Autodesk Inventor part; units mm, degrees
ref_plane "YZ Plane" through (0, 0, 0) normal (1, 0, 0) x (0, 1, 0)
ref_plane "XZ Plane" through (0, 0, 0) normal (0, 1, 0) x (-1, 0, 0)
ref_plane "XY Plane" through (0, 0, 0) normal (0, 0, 1) x (1, 0, 0)
sketch "Skizze1" plane through (0, 0, 0) normal (0, 1, 0) x (-1, 0, 0)
  circle A0 centre (0, 0) radius 27
  circle A1 centre (0, 0) radius 30
  dimension "d0" = 54
  dimension "d10" = 60
extrude "Extrusion1" add sketch "Skizze1" along normal blind 190
sketch "Skizze4" plane through (0, 0, 0) normal (0, -1, 0) x (1, 0, 0)
  circle A0 centre (0, 0) radius 30
  point P0 (0, 30)
  point P1 (-25.9808, -15)
  point P2 (25.9808, -15)
  dimension "d11" = 30
  dimension "d14" = 360
ref_plane "Arbeitsebene2" through (0, 0, 30) normal (0, 0, 1) x (1, 0, 0)
ref_plane "Arbeitsebene3" through (25.9808, 0, -15) normal (0.866, 0, -0.5) x (0, 1, 0)
ref_plane "Arbeitsebene4" through (-25.9808, 0, -15) normal (-0.866, 0, -0.5) x (0, -1, 0)
sketch "Skizze5" plane through (25.9808, 0, -15) normal (0.866, 0, -0.5) x (0, 1, 0)
  line L0 (0, 30) -> (0, -30)
  line L1 (0, 30) -> (190, 30)
  point P0 (0, 0)
  point P1 (50, 0)
  point P2 (140, 0)
  dimension "d16" = 50
  dimension "d17" = 90
  dimension "d18" = 30
  dimension "d19" = 30
sketch "Skizze6" plane through (0, 0, 30) normal (0, 0, 1) x (1, 0, 0)
  line L0 (-30, 0) -> (-30, 190)
  line L1 (-30, 0) -> (30, 0)
  point P0 (0, 0)
  point P1 (0, 20)
  point P2 (0, 110)
  dimension "d20" = 90
  dimension "d21" = 30
  dimension "d22" = 30
  dimension "d23" = 20
sketch "Skizze7" plane through (-25.9808, 0, -15) normal (-0.866, 0, -0.5) x (0, -1, 0)
  line L0 (0, 30) -> (-190, 30)
  point P0 (0, 0)
  point P1 (-80, 0)
  point P2 (-170, 0)
  dimension "d24" = 30
  dimension "d25" = 80
  dimension "d47" = 90
  dimension "d48" = 30
hole "Bohrung1" at (-25.9808, 80, -15) at (-25.9808, 170, -15) direction (0.866, 0, 0.5) diameter 3.3 depth 8 tip angle 118
hole "Bohrung2" at (0, 110, 30) at (0, 20, 30) direction (0, 0, -1) diameter 3.3 depth 8 tip angle 118
hole "Bohrung3" at (25.9808, 50, -15) at (25.9808, 140, -15) direction (-0.866, 0, 0.5) diameter 3.3 depth 8 tip angle 118
properties part number "cylinder"
Build history of the part. All positions in model axes, mm. A direction names the side the tool comes from. Give positions to 0.01 mm unless a question says otherwise; leave off trailing zeros. Order: outer loops, then holes, each group sorted by start corner. A loop starts at its lowest first (then second) coordinate and runs counter-clockwise, first axis right, second up. Notation, with made-up numbers: M -25.75,66 L -1.75,66 A16 ccw -1.75,86 Z; hole C -2.75,28 d10. An arc over 180 degrees is marked long. Use one line per item in the form item = value.
Q1. Wall check: probe 1 along Y at (x, z) = (0, 29); probe 2 along Z at (x, y) = (0, 68); probe 3 along Z at (x, y) = (6.5, 74.5). Give the ranges that are in metal, low to high.
Conclusion:
probe_1 = 0 to 18.35, 21.65 to 108.35, 111.65 to 190
probe_2 = -30 to -27, 27 to 30
probe_3 = -29.29 to -26.21, 26.21 to 29.29
Q2. Pin check, flat tips, straight feed: P1, Ø4, axis at y = 74.5, z = 9.5, coming from the +X side; P2, Ø8, axis at y = 54, z = 8, coming from the -X side; P3, Ø10, axis at y = 158, z = -16, coming from the -X side. Stop position of each tip, or through.
Conclusion:
P1 = 29.05
P2 = -29.73
P3 = -27.91
Q3. Slice it at B-B, the plane z = 17.5. Write the cut outline in (x, y).
Conclusion:
outline = M -24.37,0 L -20.56,0 L -20.56,190 L -24.37,190 Z; M 20.56,0 L 24.37,0 L 24.37,190 L 20.56,190 Z
Q4. Slice it at C-C, the plane y = 44.5. Write the cut outline in (x, z).
Conclusion:
outline = C 0,0 d60; hole C 0,0 d54
Q5. Slice it at A-A, the plane x = 11. Write the cut outline in (y, z), and give its area (3 significant figures).
Conclusion:
outline = M 0,-27.91 L 190,-27.91 L 190,-24.66 L 0,-24.66 Z; M 0,24.66 L 190,24.66 L 190,27.91 L 0,27.91 Z
area = 1,240 mm2
Q6. Pull direction X, two halves, no side cores. Call faces 1 (the flat face through (25, 0, 11)), 2 (the cylindrical face through (29.97, 93.67, -1.32)), 3 (the cylindrical face through (24.957, 141.524, -13.679)), 4 (the cylindrical face through (24.394, 51.574, -14.656)): released by +X, released by -X, zero draft, split by the parting line, or undercut.
Conclusion:
face_1 = zero draft
face_2 = split by the parting line
face_3 = undercut
face_4 = undercut
Q7. Which spindle directions (+Z, -Z, +X, -X, +Y, -Y) get a long thin tool onto all of the face, cutting with end or side? Do faces 5 (the cylindrical face through (1, 21.31, 28.45)), 6 (the cylindrical face through (-24.325, 171.524, -14.774)). Say none if no direction does.
Conclusion:
face_5 = +Z
face_6 = none
